from build123d import *

# Parameters (mm, degrees)
F1_DEPTH = 1.5
F3_DEPTH = 1.8
F4_W     = 6.4
F4_H     = 0.4
F5_DEPTH = 4
F6_DEPTH = 24


with BuildPart() as f1:
    # F0 (on Top) → F1 (new body)
    with BuildSketch(Plane.XY):
        with BuildLine():
            Line((-8.3, -10), (8.3, -10))
            ThreePointArc((8.3, -10), (8.797918, -8.797918), (10, -8.3))
            Line((10, -8.3), (10, 8.3))
            ThreePointArc((10, 8.3), (8.797918, 8.797918), (8.3, 10))
            Line((8.3, 10), (-8.3, 10))
            ThreePointArc((-8.3, 10), (-8.797918, 8.797918), (-10, 8.3))
            Line((-10, 8.3), (-10, -8.3))
            ThreePointArc((-10, -8.3), (-8.797918, -8.797918), (-8.3, -10))
        make_face()
    extrude(amount=-F1_DEPTH)

    # F2 (on face) → F3 (join)
    with BuildSketch(Plane.XY):
        with BuildLine():
            Line((-5, -9), (5, -9))
            ThreePointArc((5, -9), (5.707107, -8.707107), (6, -8))
            Line((6, -8), (6, -4.2))
            ThreePointArc((6, -4.2), (6.292893, -3.492893), (7, -3.2))
            Line((7, -3.2), (10, -3.2))
            Line((10, -3.2), (10, 3.2))
            Line((10, 3.2), (7, 3.2))
            ThreePointArc((7, 3.2), (6.292893, 3.492893), (6, 4.2))
            Line((6, 4.2), (6, 8))
            ThreePointArc((6, 8), (5.707107, 8.707107), (5, 9))
            Line((5, 9), (-5, 9))
            ThreePointArc((-5, 9), (-5.707107, 8.707107), (-6, 8))
            Line((-6, 8), (-6, 4.2))
            ThreePointArc((-6, 4.2), (-6.292893, 3.492893), (-7, 3.2))
            Line((-7, 3.2), (-10, 3.2))
            Line((-10, 3.2), (-10, -3.2))
            Line((-10, -3.2), (-7, -3.2))
            ThreePointArc((-7, -3.2), (-6.292893, -3.492893), (-6, -4.2))
            Line((-6, -4.2), (-6, -8))
            ThreePointArc((-6, -8), (-5.707107, -8.707107), (-5, -9))
        make_face()
    extrude(amount=F3_DEPTH)

    # F4 (on face) → F5 (join)
    with BuildSketch(Plane(origin=(-10, 0, 0), x_dir=(0, -1, 0), z_dir=(-1, 0, 0))):
        with Locations((0, 0.7)):
            Rectangle(F4_W, F4_H)
    extrude(amount=F5_DEPTH)

    # F4 (on face) → F6 (join)
    with BuildSketch(Plane(origin=(-10, 0, 0), x_dir=(0, -1, 0), z_dir=(-1, 0, 0))):
        with Locations((0, 0.7)):
            Rectangle(F4_W, F4_H)
    extrude(amount=-F6_DEPTH)


solid = f1.part
Verification items for the finished model (mm, model axes). A direction names the side the tool comes from. Coordinates: 2 decimals unless noted, no trailing zeros. Loops run counter-clockwise (first coordinate to the right, second up) from the corner with the lowest first, then second, coordinate; pieces in that order, holes last. Notation, with made-up numbers: (38.25, 13) -> (59.25, 13) arc R38 ccw to (59.25, 51) -> close; hole circle Ø1 at (55.5, -40). An arc over 180 degrees is marked (long way). Answer as CSV lines item,"result".
1) Cross-section at B-B, the plane x = 7.75. Record the cut outline in (y, z), then the cut area to 3 significant figures.
Found:
outline,"(-10, -1.5) -> (10, -1.5) -> (10, 0) -> (3.2, 0) -> (3.2, 1.8) -> (-3.2, 1.8) -> (-3.2, 0) -> (-10, 0) -> close"
area,"41.5 mm2"
2) Release check for a two-part mould opening along Z. For faces 5 (the flat face through (-0.1, 9.7, 0)), 6 (the flat face through (9, -3.2, 1)), 7 (the flat face through (-12, 0, 0.5)) record: +Z half, -Z half, draft (parallel to the pull), parting line (faces both ways), or undercut.
Found:
face 5,"+Z half"
face 6,"draft"
face 7,"-Z half"
3) Cross-section at D-D, the plane x = 11.25. Record the cut outline in (y, z).
Found:
outline,"(-3.2, 0.5) -> (3.2, 0.5) -> (3.2, 0.9) -> (-3.2, 0.9) -> close"
4) Depth check by flat-ended pin: pin 1 (1.4 mm diameter, centred on x = 2.5, z = 1.5, fed in from -Y); pin 2 (0.5 mm diameter, centred on y = -1.5, z = 1.5, fed in from -X); pin 3 (1 mm diameter, centred on y = 1, z = 1, fed in from +X); pin 4 (1.4 mm diameter, centred on x = -0.5, z = 1, fed in from +Y). Enter the tip coordinate at first touch or a pass-through.
Found:
pin 1,"stops at y = -9"
pin 2,"stops at x = -10"
pin 3,"stops at x = 14"
pin 4,"stops at y = 9"
5) Cross-section at A-A, the plane z = -1.2. Record the cut outline in (x, y).
Found:
outline,"(-10, -8.3) arc R1.7 cw to (-8.3, -10) -> (8.3, -10) arc R1.7 cw to (10, -8.3) -> (10, 8.3) arc R1.7 cw to (8.3, 10) -> (-8.3, 10) arc R1.7 cw to (-10, 8.3) -> close"
6) Thickness scan on L1, parallel to Z at x = 12, y = -2.75; L2, parallel to Y at x = 3.25, z = 0.9; L3, parallel to X at y = 3.75, z = -0.6. Record the ranges inside material, lowest first. Write a range as from..to.
Found:
L1,"z = 0.5..0.9"
L2,"y = -9..9"
L3,"x = -10..10"
7) Cross-section at C-C, the plane y = -0.5. Record the cut outline in (x, z).
Found:
outline,"(-14, 0.5) -> (-10, 0.5) -> (-10, -1.5) -> (10, -1.5) -> (10, 0.5) -> (14, 0.5) -> (14, 0.9) -> (10, 0.9) -> (10, 1.8) -> (-10, 1.8) -> (-10, 0.9) -> (-14, 0.9) -> close"
8) Tool access check on faces 1 (the flat face through (0, -9, 1)), 2 (the cylindrical face through (5.715, 8.699, 0.887)), 3 (the flat face through (-9, 3.2, 1)), 4 (the cylindrical face through (6.285, -3.501, 0.887)). Record the directions out of +Z, -Z, +X, -X, +Y, -Y that give a thin tool (end or side, any length) a straight path to the whole face; none if there is none.
Found:
face 1,"+Z, +X, -X, -Y"
face 2,"+Z, +X, +Y"
face 3,"+Z, -X, +Y"
face 4,"+Z, +X, -Y"
